Build history of the part. All positions in model axes, mm. A direction names the side the tool comes from. Coordinates: 2 decimals unless noted, no trailing zeros. Write each loop counter-clockwise with the first axis right and the second up, starting at its lowest first coordinate (ties: lowest second). Pieces come first, ordered by that corner, then holes. Notation, with made-up numbers: M 67,66.5 L 93,66.5 A26 ccw 93,80.5 Z; hole C 20.25,-35 d10. An arc over 180 degrees is marked long. Use CSV: the item, a comma, the result in double quotes. Start each with the question number.
Autodesk Inventor part; units mm, degrees
ref_plane "Work Plane2" through (178, -56.0619, -70.2985) normal (1, 0, 0) x (0, 0.8411785, -0.5407576)
ref_plane "YZ Plane" through (0, 0, 0) normal (1, 0, 0) x (0, 1, 0)
ref_plane "XZ Plane" through (0, 0, 0) normal (0, 1, 0) x (-1, 0, 0)
ref_plane "Work Plane1" through (0, 4.7283, -22.9522) normal (-1, 0, 0) x (0, -0.8411785, 0.5407576)
sketch "Sketch1" plane through (0, 4.7283, -22.9522) normal (-1, 0, 0) x (0, -0.8411785, 0.5407576)
  line L0 (-34.301, -16.75) -> (61.5, -16.75)
  line L1 (61.5, -16.75) -> (61.5, -12.25)
  line L2 (61.5, -12.25) -> (16.3889, 16.75)
  line L3 (16.3889, 16.75) -> (-61.5, 16.75)
  line L4 (-61.5, 16.75) -> (-61.5, -12.801)
  line L5 (61.5, -12.25) -> (61.5, -16.75)
  line L6 (61.5, -16.75) -> (65.5, -16.75)
  line L7 (65.5, -16.75) -> (65.5, -20.25)
  line L8 (65.5, -20.25) -> (79.5, -20.25)
  line L9 (79.5, -20.25) -> (65.5, -11.25)
  line L10 (65.5, -11.25) -> (65.5, -12.25)
  line L11 (65.5, -12.25) -> (61.5, -12.25)
  line L12 (16.3889, 16.75) -> (16.3889, 18.75)
  line L13 (14.3494, 18.75) -> (16.3889, 18.75)
  line L14 (65.3834, -12.25) -> (12.6747, 21.6342)
  line L15 (16.3889, 16.75) -> (16.3889, 19.2465)
  arc A0 (-57.551, -16.75) -> (-61.5, -12.801) centre (-58.75, -14) ccw
  line L16 (-57.551, -16.75) -> (-36.699, -16.75)
  arc A1 (-34.301, -16.75) -> (-36.699, -16.75) centre (-35.5, -14) ccw
  dimension "d13" = 2.1
ref_plane "Work Plane2" through (178, -56.0619, -70.2985) normal (1, 0, 0) x (0, 0.8411785, -0.5407576)
extrude "Extrusion1" add sketch "Sketch1" against normal up to surface (178 mm away) contours L2 L12 L15 L14 L11
sketch "Sketch2" plane through (0, -56.8951, 2.1) normal (0, 0, 1) x (1, 0, 0)
  circle A0 centre (3, 22.9238) radius 2.5
  circle A1 centre (3, 42.238) radius 2.5
  line L0 (0, 3.2667) -> (0, 56.8951)
  line L1 (0, 3.2667) -> (6, 3.2667)
  line L2 (6, 56.8951) -> (6, 3.2667)
  line L3 (0, 56.8951) -> (6, 56.8951)
  circle A2 centre (175, 22.9238) radius 2.5
  circle A3 centre (175, 42.238) radius 2.5
  line L4 (178, 3.2667) -> (178, 56.8951)
  line L5 (178, 56.8951) -> (172, 56.8951)
  line L6 (172, 56.8951) -> (172, 3.2667)
  line L7 (178, 3.2667) -> (172, 3.2667)
hole "Hole1" at (3, -14.6571, 2.1) at (3, -33.9713, 2.1) at (175, -33.9713, 2.1) at (175, -14.6571, 2.1) direction (0, 0, -1) diameter 3.6 end through all countersink diameter 7 countersink angle 90
ref_plane "Work Plane3" through (22, -30.5397, -9.0869) normal (0, -0.7712334, 0.6365525) x (1, 0, 0)
sketch "Sketch3" plane through (22, -30.5397, -9.0869) normal (0, -0.7712334, 0.6365525) x (1, 0, 0)
  line L0 (-9.9215, 5.4518) -> (-9.9215, -5.4534)
  spline S0 degree 3 poles (-9.9215, -5.4534) (-9.9222, -5.5772) (-9.8204, -5.8209) (-9.5772, -5.9222) (-9.4534, -5.9215) knots 0 0 0 0 0.5 1 1 1 1
  line L1 (-9.4534, -5.9215) -> (19.4534, -5.9215)
  spline S1 degree 3 poles (19.4534, -5.9215) (19.5775, -5.9222) (19.8219, -5.82) (19.9222, -5.5758) (19.9215, -5.4518) knots 0 0 0 0 0.5 1 1 1 1
  line L2 (19.9215, -5.4518) -> (19.9215, 5.4534)
  spline S2 degree 3 poles (19.9215, 5.4534) (19.9222, 5.5775) (19.82, 5.8219) (19.5758, 5.9222) (19.4518, 5.9215) knots 0 0 0 0 0.5 1 1 1 1
  line L3 (19.4518, 5.9215) -> (-9.4534, 5.9215)
  spline S3 degree 3 poles (-9.4534, 5.9215) (-9.5775, 5.9222) (-9.8219, 5.82) (-9.9222, 5.5758) (-9.9215, 5.4518) knots 0 0 0 0 0.5 1 1 1 1
  circle A0 centre (-8.3791, -4.3791) radius 0.5
  circle A1 centre (-8.3791, 4.3791) radius 0.5
  circle A2 centre (18.3791, 4.3791) radius 0.5
  circle A3 centre (18.3791, -4.3791) radius 0.5
  arc A4 (5.2617, -1.4512) -> (5.1811, -1.5218) centre (5.2771, -1.55) ccw
  arc A5 (5.1811, 1.5218) -> (5.1811, -1.5218) centre (0, 0) ccw
  arc A6 (5.1811, 1.5218) -> (5.2617, 1.4512) centre (5.2771, 1.55) ccw
  arc A7 (5.2617, 1.4512) -> (5.3414, 1.519) centre (5.2463, 1.55) ccw
  arc A8 (5.3414, -1.519) -> (5.3414, 1.519) centre (10, 0) ccw
  arc A9 (5.3414, -1.519) -> (5.2617, -1.4512) centre (5.2463, -1.55) ccw
  line L4 (143.9215, 5.4518) -> (143.9215, -5.4534)
  spline S4 degree 3 poles (143.4534, 5.9215) (143.5775, 5.9222) (143.8219, 5.82) (143.9222, 5.5758) (143.9215, 5.4518) knots 0 0 0 0 0.5 1 1 1 1
  line L5 (114.5482, 5.9215) -> (143.4534, 5.9215)
  spline S5 degree 3 poles (114.0785, 5.4534) (114.0778, 5.5775) (114.18, 5.8219) (114.4242, 5.9222) (114.5482, 5.9215) knots 0 0 0 0 0.5 1 1 1 1
  line L6 (114.0785, -5.4518) -> (114.0785, 5.4534)
  spline S6 degree 3 poles (114.5466, -5.9215) (114.4225, -5.9222) (114.1781, -5.82) (114.0778, -5.5758) (114.0785, -5.4518) knots 0 0 0 0 0.5 1 1 1 1
  line L7 (143.4534, -5.9215) -> (114.5466, -5.9215)
  spline S7 degree 3 poles (143.9215, -5.4534) (143.9222, -5.5772) (143.8204, -5.8209) (143.5772, -5.9222) (143.4534, -5.9215) knots 0 0 0 0 0.5 1 1 1 1
  circle A10 centre (142.3791, -4.3791) radius 0.5
  circle A11 centre (142.3791, 4.3791) radius 0.5
  circle A12 centre (115.6209, 4.3791) radius 0.5
  circle A13 centre (115.6209, -4.3791) radius 0.5
  arc A14 (128.8189, -1.5218) -> (128.7383, -1.4512) centre (128.7229, -1.55) ccw
  arc A15 (128.7383, -1.4512) -> (128.6586, -1.519) centre (128.7537, -1.55) ccw
  arc A16 (128.6586, 1.519) -> (128.6586, -1.519) centre (124, 0) ccw
  arc A17 (128.6586, 1.519) -> (128.7383, 1.4512) centre (128.7537, 1.55) ccw
  arc A18 (128.7383, 1.4512) -> (128.8189, 1.5218) centre (128.7229, 1.55) ccw
  arc A19 (128.8189, -1.5218) -> (128.8189, 1.5218) centre (134, 0) ccw
  circle A20 centre (10, 0) radius 5.4
  circle A21 centre (124, 0) radius 5.4
  line L8 (0, 5.4) -> (10, 5.4)
  line L9 (10, -5.4) -> (0, -5.4)
  line L10 (124, 5.4) -> (134, 5.4)
  line L11 (134, -5.4) -> (124, -5.4)
  point P0 (-22, 26.4483)
  dimension "d9" = 10.8
  dimension "d10" = 10.8
extrude "Extrusion2" cut sketch "Sketch3" along normal blind 78.25 contours A9 A8 A7 A6 A5 A20 A4 | A4 A5 A20 A6 A7 A8 A9 | A20 L9 A5 | A5 A20 | A5 L8 A20 | A19 A21 A18 A17 A16 A15 A14 | A14 A15 A16 A17 A18 A19 A21 | A21 A19 | A19 L11 A21 | A19 A21 L10
properties part number "front"
1. Slice it at B-B (x = 144.5). List the corners of the cut face in (y, z), and give its area (3 significant figures).
2. Slice it at C-C (y = -47). Count the separate pieces of the cut face and the enclosed holes in it, and give its area (3 significant figures).
3. Pull direction X, two halves, no side cores. Call faces 1 (the cylindrical face through (176.6, -34.8, 0.2)), 2 (the flat face through (88, -28, 2.1)): pulls with the +X half, pulls with the -X half, needs draft (parallel to the pull), parting line crosses it, or undercut.
4. Flat gauge pins, fed straight in: pin 1 (6 mm diameter, centred on x = 175, y = -33.97, fed in from +Z); pin 2 (4.5 mm diameter, centred on x = 3, y = -33.97, fed in from +Z). Where does each tip first touch, or does it go through?
5. Drill centre lines: line 1 along Y through (x, z) = (3, 0.2); line 2 along X through (y, z) = (-43, 0.65); line 3 along X through (y, z) = (-41, 1.4). Where is each one in solid material? Low to high. Write a range as from..to.
6. 3-axis set-ups, long thin cutter, end or side, ignore diameter. For faces 3 (the cylindrical face through (16.64, -43.22, 0.51)), 4 (the cylindrical face through (2.459, -16.374, 0.197)): which of +Z, -Z, +X, -X, +Y, -Y reach the whole face in a straight line?
7. Slice it at A-A (x = 175). List the corners of the cut face in (y, z), and give its area (3 significant figures).
Established:
1,outline,"M -56.9,2.1 L -53.63,0 L -49.7,0 L -52.24,2.1 Z; M -35.94,2.1 L -33.4,0 L 0,0 L 1.35,2.1 Z"
1,area,"83.2 mm2"
2,separate pieces,"3"
2,enclosed holes,"0"
2,area,"293 mm2"
3,face 1,"undercut"
3,face 2,"needs draft"
4,pin 1,"stops at z = 1.6"
4,pin 2,"stops at z = 0.85"
5,line 1,"y = -53.94..-35.77, -32.17..-16.46, -12.86..0.13"
5,line 2,"x = 0..16.62, 37.38..140.62, 161.38..178"
5,line 3,"x = 0..16.79, 37.21..140.79, 161.21..178"
6,face 3,"none"
6,face 4,"+Z, -Z"
7,outline,"M -56.9,2.1 L -53.63,0 L -35.77,0 L -35.77,0.4 L -37.47,2.1 Z; M -32.17,0 L -16.46,0 L -16.46,0.4 L -18.16,2.1 L -30.47,2.1 L -32.17,0.4 Z; M -12.86,0 L 0,0 L 1.35,2.1 L -11.16,2.1 L -12.86,0.4 Z"
7,area,"96.6 mm2"
